from build123d import *

# Parameters (mm, degrees)
PAD_DEPTH       = 5
FILLET_R        = 4
POCKET_DEPTH    = 2
SKETCH011_R     = 1.6
POCKET001_DEPTH = 5
SKETCH012_R     = 3
POCKET002_DEPTH = 3.5


with BuildPart() as pocket002:
    # Sketch010 → Pad (new body)
    with BuildSketch(Plane.XY):
        with BuildLine():
            Line((44.86111, -50), (59.975919, -16.416677))
            ThreePointArc((59.975919, -16.416677), (62.609058, -8.395333), (63.5, 0))
            Line((57.7, 0), (63.5, 0))
            ThreePointArc((51.3, 0), (54.5, -3.2), (57.7, 0))
            Line((0, 0), (51.3, 0))
            Line((0, -53.373162), (0, 0))
            ThreePointArc((0, -53.373162), (22.493874, -52.528683), (44.86111, -50))
        make_face()
    extrude(amount=-PAD_DEPTH)

    # Fillet
    fillet_edges = [pocket002.edges().sort_by_distance(p)[0] for p in [
        (44.86111, -50, -2.5),
    ]]
    fillet(fillet_edges, radius=FILLET_R)

    # Sketch (on Face5 of Fillet) → Pocket (cut)
    with BuildSketch(Plane(origin=(0, 0, -5), x_dir=(1, 0, 0), z_dir=(0, 0, -1))):
        with BuildLine():
            ThreePointArc((42.691795, 48.319977), (21.400417, 50.608892), (0, 51.373162))
            Line((0, 0), (0, 51.373162))
            Line((49.3, 0), (0, 0))
            ThreePointArc((57.658949, 4.130502), (52.196365, 4.661895), (49.3, 0))
            ThreePointArc((57.658949, 4.130502), (59.892731, 3.998098), (60.851148, 6.020164))
            ThreePointArc((60.851148, 6.020164), (59.670721, 11.322874), (57.782667, 16.416731))
            Line((57.782667, 16.416731), (49.614632, 34.565141))
            ThreePointArc((49.614632, 34.565141), (48.503106, 35.613174), (46.975994, 35.570785))
            ThreePointArc((43.16421, 44.48914), (40.540272, 38.093872), (46.975994, 35.570785))
            ThreePointArc((43.16421, 44.48914), (44.392147, 46.585115), (42.691795, 48.319977))
        make_face()
    extrude(amount=-POCKET_DEPTH, mode=Mode.SUBTRACT)

    # Sketch011 (on Face5 of Pocket) → Pocket001 (cut)
    with BuildSketch(Plane(origin=(0, 0, -5), x_dir=(1, 0, 0), z_dir=(0, 0, -1))):
        with Locations((45, 40)):
            Circle(SKETCH011_R)
    extrude(amount=-POCKET001_DEPTH, mode=Mode.SUBTRACT)

    # Sketch012 (on Face5 of Pocket001) → Pocket002 (cut)
    with BuildSketch(Plane(origin=(0, 0, -5), x_dir=(1, 0, 0), z_dir=(0, 0, -1))):
        with Locations((45, 40)):
            Circle(SKETCH012_R)
    extrude(amount=-POCKET002_DEPTH, mode=Mode.SUBTRACT)


with BuildPart() as fusion:
    # Part__Mirroring: instance of Pocket002
    add(pocket002.part.mirror(Plane(origin=(0, 0, 0), x_dir=(1, 0, 0), z_dir=(0, 1, 0))))

    # Fusion: union Pocket002
    add(pocket002.part)


with BuildPart() as fusion005:
    # Part__Mirroring001: instance of Fusion
    add(fusion.part.mirror(Plane(origin=(0, 0, 0), x_dir=(0, -1, 0), z_dir=(1, 0, 0))))

    # Fusion005: union Fusion
    add(fusion.part)


solid = fusion005.part
For this review, take the finished solid that the model builds, in its own axes (mm). A direction names the side the tool comes from. Coordinates: 2 decimals unless noted, no trailing zeros. Loops run counter-clockwise (first coordinate to the right, second up) from the corner with the lowest first, then second, coordinate; pieces in that order, holes last. Notation, with made-up numbers: (-4, -19.5) - (14, -19.5) arc R16 ccw to (14, -0.5) - close; hole circle Ø5 at (77.5, 85.25). An arc over 180 degrees is marked (long way). Use a Markdown table: item, result. Add a question column.
Item 1: We need section A-A (x = -54.5). Give the boundary of the cut face in (y, z), and give its area (3 significant figures).
Item 2: For line 1 (Y direction, x = 0, z = -3.8); line 2 (Y direction, x = 45, z = -0.7); line 3 (Z direction, x = -48, y = 17), list the stretches that pass through material, from the lowest coordinate up.
Item 3: Mouldability with a two-part tool opening along Y and no side actions: class faces 3 (the face through (42.79, 42.03, -3.27)), 4 (the face through (-44.54, -49.54, -2.54)), 5 (the face through (-1, 1, 0)) as pulls with the +Y half, pulls with the -Y half, needs draft (parallel to the pull), parting line crosses it, or undercut.
Item 4: Tool access review of faces 1 (the face through (45.74, 38.58, -0.76)), 2 (the face through (59.692, -11.25, -4.014)): name each direction out of +Z, -Z, +X, -X, +Y, -Y from which nothing blocks a thin tool from reaching the whole face with its end or side.
Item 5: Insertion check: pin 1 Ø1.8 at (x, y) = (-44.5, 38.5) entering from -Z; pin 2 Ø3 at (y, z) = (-37, -3) entering from +X; pin 3 Ø3 at (x, y) = (-45, -40) entering from -Z; pin 4 Ø10 at (x, y) = (-48.5, -18) entering from -Z. Each pin has a flat end and moves straight along its axis. Give the tip position at first contact, or say it passes through.
Item 6: We need section B-B (y = -40). Give the boundary of the cut face in (x, z).
Item 7: We need section C-C (x = -10.5). Give the boundary of the cut face in (y, z).
Item 8: We need section D-D (y = 27). Give the boundary of the cut face in (x, z).
Results list:
| question | item | result |
|---|---|---|
| 1 | outline | (-28.58, -5) - (-23.71, -5) - (-23.71, -3) - (-5.2, -3) - (-5.2, -5) - (-3.2, -5) - (-3.2, 0) - (-28.58, 0) - close; (3.2, -5) - (5.2, -5) - (5.2, -3) - (23.71, -3) - (23.71, -5) - (28.58, -5) - (28.58, 0) - (3.2, 0) - close |
| 1 | area | 180 mm^2 |
| 2 | line 1 | y = -53.37 to -51.37, 51.37 to 53.37 |
| 2 | line 2 | y = -49.13 to -41.6, -38.4 to 38.4, 41.6 to 49.13 |
| 2 | line 3 | z = -3 to 0 |
| 3 | face 3 | undercut |
| 3 | face 4 | pulls with the -Y half |
| 3 | face 5 | needs draft |
| 4 | face 1 | +Z, -Z |
| 4 | face 2 | -Z |
| 5 | pin 1 | stops at z = -1.5 |
| 5 | pin 2 | stops at x = 51.39 |
| 5 | pin 3 | passes through |
| 5 | pin 4 | stops at z = -3 |
| 6 | outline | (-49.36, -5) - (-48, -5) - (-48, -1.5) - (-46.6, -1.5) - (-46.6, 0) - (-49.36, 0) - close; (-43.4, -1.5) - (-42, -1.5) - (-42, -5) - (-40.15, -5) - (-40.15, -3) - (40.15, -3) - (40.15, -5) - (42, -5) - (42, -1.5) - (43.4, -1.5) - (43.4, 0) - (-43.4, 0) - close; (46.6, -1.5) - (48, -1.5) - (48, -5) - (49.36, -5) - (49.36, 0) - (46.6, 0) - close |
| 7 | outline | (-53.19, -5) - (-51.19, -5) - (-51.19, -3) - (51.19, -3) - (51.19, -5) - (53.19, -5) - (53.19, 0) - (-53.19, 0) - close |
| 8 | outline | (-55.21, -5) - (-53.02, -5) - (-53.02, -3) - (53.02, -3) - (53.02, -5) - (55.21, -5) - (55.21, 0) - (-55.21, 0) - close |
